Autodesk Inventor part; units mm, degrees
ref_plane "YZ Plane" through (0, 0, 0) normal (1, 0, 0) x (0, 1, 0)
ref_plane "XZ Plane" through (0, 0, 0) normal (0, 1, 0) x (-1, 0, 0)
ref_plane "XY Plane" through (0, 0, 0) normal (0, 0, 1) x (1, 0, 0)
sketch "Sketch1" plane through (0, 0, 0) normal (0, 0, 1) x (1, 0, 0)
  circle A0 centre (-24.4499, 7.2424) radius 7.5
  circle A1 centre (18.497, 17.553) radius 7.5
  circle A2 centre (5.9529, -24.7954) radius 7.5
  circle A3 centre (0, 0) radius 40
  circle A4 centre (0, 0) radius 41.25
  point P0 (0, 0)
  dimension "d9" = 82.5
extrude "Extrusion1" add sketch "Sketch1" against normal blind 20 contours A3 | A4
sketch "Sketch4" plane through (0, 0, -20) normal (0, 0, -1) x (-1, 0, 0)
  circle A0 centre (0, 0) radius 41.25
  circle A1 centre (0, 0) radius 40
  point P0 (0, 0)
  dimension "d10" = 80
extrude "Extrusion4" cut sketch "Sketch4" against normal blind 10 contours A1
properties part number "Cover of gearbox 2"
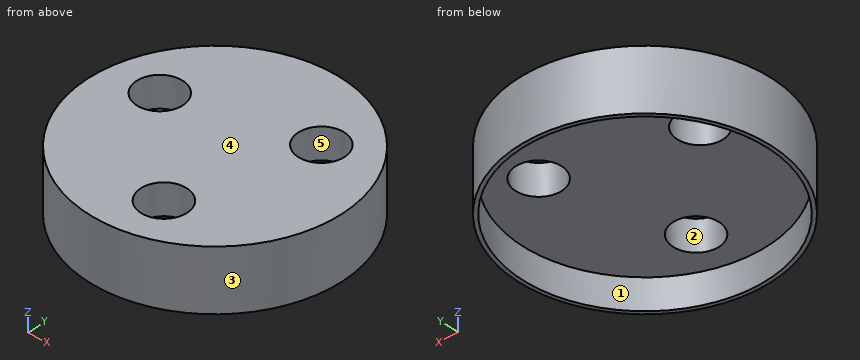
Here's how the part is built. I have some questions about the finished solid (model axes, mm). Face numbers are marked on the shaded views. A direction names the side the tool comes from. Coordinates: 2 decimals unless noted, no trailing zeros. Write each loop counter-clockwise with the first axis right and the second up, starting at its lowest first coordinate (ties: lowest second). Pieces come first, ordered by that corner, then holes. Notation, with made-up numbers: (16, 18) -> (47, 18) arc R16 cw to (47, 47) -> close; hole circle Ø1 at (-1.75, -32.5). An arc over 180 degrees is marked (long way). Use a Markdown table: item, result. Add a question column.
(1) Please list where these lines run through material, in increasing order: line 1 (Z direction, x = 17.5, y = -3); line 2 (X direction, y = 1, z = -16); line 3 (X direction, y = 12.5, z = -4.25).
(2) I'm going to push flat-ended pins straight in: P1, Ø1.5, axis at y = 23.5, z = -4, coming from the -X side; P2, Ø1.5, axis at x = -26.5, z = -5, coming from the +Y side; P3, Ø2, axis at x = -12, z = -3, coming from the +Y side. Where does each tip first touch, or does it pass through?
(3) We'd pull the mould along X, two halves only. Please class the marked faces 3, 4 and 5: +X half, -X half, draft (parallel to the pull), parting line (faces both ways), or undercut.
(4) For the marked faces 1 and 2, which set-ups out of +Z, -Z, +X, -X, +Y, -Y let a thin tool reach every point of the face, with its end or its side?
(5) If we section it at D-D, the plane y = -4.5: Write out the boundary of the cut face in (x, z).
(6) If we section it at B-B, the plane z = -16.75: Write out the boundary of the cut face in (x, y), and give its area (3 significant figures).
(7) If we section it at C-C, the plane x = 24: Write out the boundary of the cut face in (y, z).
(8) If we section it at A-A, the plane x = 0: Write out the boundary of the cut face in (y, z), and give its area (3 significant figures).
Outcome:
| question | item | result |
|---|---|---|
| 1 | line 1 | z = -10 to 0 |
| 1 | line 2 | x = -41.24 to -39.99, 39.99 to 41.24 |
| 1 | line 3 | x = -39.31 to -29.8, -19.1 to 12.95, 24.04 to 39.31 |
| 2 | P1 | stops at x = -34.41 |
| 2 | P2 | stops at y = 32.23 |
| 2 | P3 | stops at y = 39.76 |
| 3 | face 3 | parting line |
| 3 | face 4 | draft |
| 3 | face 5 | undercut |
| 4 | face 1 | -Z |
| 4 | face 2 | +Z, -Z |
| 5 | outline | (-41, -20) -> (-39.75, -20) -> (-39.75, -10) -> (39.75, -10) -> (39.75, -20) -> (41, -20) -> (41, 0) -> (-41, 0) -> close |
| 6 | outline | circle Ø82.5 at (0, 0); hole circle Ø80 at (0, 0) |
| 6 | area | 319 mm^2 |
| 7 | outline | (-33.55, -20) -> (-32, -20) -> (-32, -10) -> (12.46, -10) -> (12.46, 0) -> (-33.55, 0) -> close; (22.65, -10) -> (32, -10) -> (32, -20) -> (33.55, -20) -> (33.55, 0) -> (22.65, 0) -> close |
| 8 | outline | (-41.25, -20) -> (-40, -20) -> (-40, -10) -> (-29.36, -10) -> (-29.36, 0) -> (-41.25, 0) -> close; (-20.23, -10) -> (40, -10) -> (40, -20) -> (41.25, -20) -> (41.25, 0) -> (-20.23, 0) -> close |
| 8 | area | 759 mm^2 |
